from build123d import *

# Parameters (mm, degrees)
BOSS_EXTRUDE1_DEPTH = 6.35
SKETCH2_R           = 85
CUT_EXTRUDE1_DEPTH  = 6.35
FILLET1_R           = 60
CUT_EXTRUDE2_DEPTH  = 6.35
FILLET2_R           = 20


with BuildPart() as part:
    # Sketch1 → Boss-Extrude1 (new body)
    with BuildSketch(Plane(origin=(0, 0, 0), x_dir=(1, 0, 0), z_dir=(0, 1, 0))):
        Polygon((0, 0), (-350, -606.217782649), (350, -606.217782649), align=None)
    extrude(amount=BOSS_EXTRUDE1_DEPTH)

    # Sketch2 → Cut-Extrude1 (cut)
    with BuildSketch(Plane(origin=(0, 6.35, 0), x_dir=(1, 0, 0), z_dir=(0, 1, 0))):
        with Locations(Location((0, -404.145188433, 0), (0, 0, 270))):
            Circle(SKETCH2_R)
    extrude(amount=-CUT_EXTRUDE1_DEPTH, mode=Mode.SUBTRACT)

    # Fillet1
    fillet1_edges = [part.edges().sort_by_distance(p)[0] for p in [
        (350, 3.175, 606.217782649),
        (-350, 3.175, 606.217782649),
        (0, 3.175, 0),
    ]]
    fillet(fillet1_edges, radius=FILLET1_R)

    # Sketch3 → Cut-Extrude2 (cut)
    with BuildSketch(Plane(origin=(0, 6.35, 0), x_dir=(1, 0, 0), z_dir=(0, 1, 0))):
        with BuildLine():
            Line((30.480762114, -411.350959799), (21.480762114, -426.939417067))
            add(Edge.make_bspline(
                [(30.480762114, -411.350959799), (545.596004384, -719.145188433), (21.480762114, -426.939417067)],
                knots=[0, 0, 0, 1, 1, 1], degree=2, weights=[1, 0.290322581, 1]))
        make_face()
        with BuildLine():
            Line((-9, -374.145188433), (9, -374.145188433))
            add(Edge.make_bspline(
                [(-9, -374.145188433), (0, 225.854811567), (9, -374.145188433)],
                knots=[0, 0, 0, 1, 1, 1], degree=2, weights=[1, 0.290322581, 1]))
        make_face()
        with BuildLine():
            Line((-21.480762114, -426.939417067), (-30.480762114, -411.350959799))
            add(Edge.make_bspline(
                [(-21.480762114, -426.939417067), (-545.596004384, -719.145188433), (-30.480762114, -411.350959799)],
                knots=[0, 0, 0, 1, 1, 1], degree=2, weights=[1, 0.290322581, 1]))
        make_face()
    extrude(amount=-CUT_EXTRUDE2_DEPTH, mode=Mode.SUBTRACT)

    # Fillet2
    fillet2_edges = [part.edges().sort_by_distance(p)[0] for p in [
        (-7.677401055, 3.175, 319.492618991),
        (7.677401055, 3.175, 319.492618991),
        (77.149976159, 3.175, 439.822648805),
        (69.472575104, 3.175, 453.120297502),
        (-69.472575104, 3.175, 453.120297502),
        (-77.149976159, 3.175, 439.822648805),
    ]]
    fillet(fillet2_edges, radius=FILLET2_R)


solid = part.part
Build history of the part. All positions in model axes, mm. A direction names the side the tool comes from. Coordinates: 2 decimals unless noted, no trailing zeros. Order: outer loops, then holes, each group sorted by start corner. A loop starts at its lowest first (then second) coordinate and runs counter-clockwise, first axis right, second up. Notation, with made-up numbers: (86.25, 45) - (115.25, 45) arc R26 ccw to (115.25, 71) - close; hole circle Ø9 at (47.5, 80). An arc over 180 degrees is marked (long way). Write item = value, one per line. Start each with the question number.
1) Saw through at A-A on z = 377.5. Write the cut outline in (x, y).
2) Saw through at D-D on z = 188.5. Write the cut outline in (x, y).
3) Flat gauge pins, fed straight in: pin 1 Ø3 at (y, z) = (2.5, 158.5) entering from +X; pin 2 Ø2 at (y, z) = (0.5, 209) entering from +X. Where does each tip first touch, or does it go through?
4) Saw through at B-B on z = 475. Count the separate pieces of the cut face and the enclosed holes in it, then the cut area to 3 significant figures.
5) Two-plate mould, pull along Z, no slides. Class faces 1 (the face through (-73.14, 3.22, 360.84)), 2 (the face through (-72, 0, 329)), 3 (the face through (176.72, 3.13, 306.09)): pulls with the +Z half, pulls with the -Z half, needs draft (parallel to the pull), parting line crosses it, or undercut.
6) Saw through at C-C on x = -204.5. Write the cut outline in (y, z).
7) 3-axis set-ups, long thin cutter, end or side, ignore diameter. For faces 4 (the face through (-298.473, 3.219, 575.453)), 5 (the face through (74.1, 3.2, 362.5)): which of +Z, -Z, +X, -X, +Y, -Y reach the whole face in a straight line?
8) Wall check: line 1 along X through (y, z) = (0.5, 472.5); line 2 along X through (y, z) = (6, 397); line 3 along Z through (x, y) = (-25, 2.25). Give the ranges that are in metal, low to high. Write a range as from..to.
From the geometry:
q1.outline = (-217.95, 0) - (-80.72, 0) - (-80.72, 6.35) - (-217.95, 6.35) - close; (80.72, 0) - (217.95, 0) - (217.95, 6.35) - (80.72, 6.35) - close
q2.outline = (-108.83, 0) - (108.83, 0) - (108.83, 6.35) - (-108.83, 6.35) - close
q3.pin_1 = 92.38
q3.pin_2 = 121.24
q4.separate_pieces = 4
q4.enclosed_holes = 0
q4.area = 2,660 mm^2
q5.face_1 = undercut
q5.face_2 = needs draft
q5.face_3 = pulls with the -Z half
q6.outline = (0, 354.2) - (6.35, 354.2) - (6.35, 606.22) - (0, 606.22) - close
q7.face_4 = -X, +Y, -Y
q7.face_5 = +Y, -Y
q8.line_1 = -272.8..-126.96, -107.11..-50.52, 50.52..107.11, 126.96..272.8
q8.line_2 = -229.21..-84.7, 84.7..229.21
q8.line_3 = 65.46..322.9, 485.39..606.22
